The model under review builds one solid part; all positions refer to its coordinate system, in mm. Coordinates: 2 decimals unless noted, no trailing zeros. Loops run counter-clockwise (first coordinate to the right, second up) from the corner with the lowest first, then second, coordinate; pieces in that order, holes last. Notation, with made-up numbers: (17, -3) - (22, -3) arc R16 cw to (22, 1) - close; hole circle Ø5 at (-37, -26.75). An arc over 180 degrees is marked (long way). One line per item, written item: value. Start each with the question number.
1. To check wall thickness, follow line 1 (X direction, y = 5, z = -78); line 2 (X direction, y = 10, z = -102); line 3 (Z direction, x = -147, y = 33). State the ranges of each line that lie inside material, in increasing order.
2. We need section B-B, the plane z = -111. Give the boundary of the cut face in (x, y).
3. We need section A-A, the plane x = -156.5. Give the boundary of the cut face in (y, z).
4. We need section C-C, the plane z = -180. Give the boundary of the cut face in (x, y).
5. Insertion check: P1, Ø2, axis at x = 0.5, y = 3, coming from the +Z side; P2, Ø4, axis at x = 67.5, y = 18.5, coming from the +Z side; P3, Ø3, axis at x = 261.5, y = 23.5, coming from the +Z side. Each pin has a flat end and moves straight along its axis. Give the tip position at first contact, or say it passes through.
from build123d import *

# Parameters (mm, degrees)
BARRER1_PROFILE_R = 15


with BuildPart() as part:
    # Barrer1: sweep along a curve in space
    with BuildLine() as barrer1_path:
        Line((264.918926477, 18.063618937, 18.063618937), (226.035142661, 27.418597771, 27.418597771))
        ThreePointArc((226.035142661, 27.418597771, 27.418597771), (210.148674123, 30.238757749, 30.238757749), (193.824243162, 31.187293721, 31.187293721))
        Line((193.824243162, 31.187293721, 31.187293721), (-193.824243162, 31.187293721, 31.187293721))
        ThreePointArc((-193.824243162, 31.187293721, 31.187293721), (-210.148674123, 30.238757749, 30.238757749), (-226.035142661, 27.418597771, 27.418597771))
        Line((-264.918926477, 18.063618937, 18.063618937), (-226.035142661, 27.418597771, 27.418597771))
        ThreePointArc((-264.918926477, 18.063618937, 18.063618937), (-318.95127781, 5.064073793, -17.169648176), (-340, 0, -79.30798358))
        Line((-340, 0, -79.30798358), (-340, 0, -180))
        Line((-340, 0, -180), (340, 0, -180))
        Line((340, 0, -79.30798358), (340, 0, -180))
        ThreePointArc((264.918926477, 18.063618937, 18.063618937), (318.95127781, 5.064073793, -17.169648176), (340, 0, -79.30798358))
    # Barrer1 profile (on start of the path) → Barrer1 (sweep)
    with BuildSketch(Plane(origin=(264.918926477, 18.063618937, 18.063618937), x_dir=(-0.23391363473017787, 0, -0.9722573792403516), z_dir=(-0.9467025907554608, 0.22776545464237832, 0.22776545464237832))):
        Circle(BARRER1_PROFILE_R)
    sweep(path=barrer1_path.line, transition=Transition.RIGHT)


solid = part.part
Findings below:
1. line 1: -354.14 to -325.85, 325.85 to 354.14
1. line 2: -351.18 to -328.82, 328.82 to 351.18
1. line 3: 16.3 to 46.08
2. outline: circle Ø30 at (-340, 0); circle Ø30 at (340, 0)
3. outline: circle Ø30 at (0, -180); circle Ø30 at (31.19, 31.19)
4. outline: (-340, -15) - (340, -15) arc R15 ccw to (340, 15) - (-340, 15) arc R15 ccw to start
5. P1: z = -165.13
5. P2: z = 41.71
5. P3: z = 34.38
